Check sheet for the modelled part. Datum: model origin and axes. Units: mm. A direction names the side the tool comes from. Give positions to 0.01 mm unless a question says otherwise; leave off trailing zeros. Write each loop counter-clockwise with the first axis right and the second up, starting at its lowest first coordinate (ties: lowest second). Pieces come first, ordered by that corner, then holes. Notation, with made-up numbers: M 4.5,85 L 44.5,85 A15 cw 44.5,90 Z; hole C 78,-8 d4. An arc over 180 degrees is marked long. Use CSV: the item, a comma, the result in double quotes. Start each with the question number.
1. Cross-section at D-D, the plane x = 5.5. Enter the section's corners in (y, z).
2. Access from +Z, -Z, +X, -X, +Y, -Y to the whole of each face (thin tool, end or side, straight path). Record for faces 1 (the face through (-6, 10, -2)), 2 (the face through (0, 3, -2.975)), 3 (the face through (2.975, 3, 0)), 4 (the face through (0, 3, 2.975)), 5 (the face through (-2.777, 7.972, 6.697)).
3. Depth check by flat-ended pin: P1, Ø4.5, axis at x = 3, z = 0, coming from the -Y side; P2, Ø1.7, axis at x = 0, z = 0, coming from the -Y side; P3, Ø4, axis at y = 9.5, z = 4.5, coming from the -X side; P4, Ø4, axis at x = -3.5, y = 3, coming from the +Z side (3 decimals). Enter the tip coordinate at first touch or a pass-through.
4. Cross-section at C-C, the plane z = -5. Enter the section's corners in (x, y).
5. Cross-section at B-B, the plane x = -0.25. Enter the section's corners in (y, z) (3 decimals), and give its area (3 significant figures).
6. Cross-section at A-A, the plane y = 3.75. Enter the section's corners in (x, z) (3 decimals).
7. Scan lines: line 1 (Z direction, x = 0, y = 3.25) (3 decimals); line 2 (X direction, y = 8, z = 0) (3 decimals). Record each from-to range of solid material in increasing order.
8. Mould release check, pull along X, two halves, no side actions. Record for faces 6 (the face through (0, 12.2, -5.5)), 7 (the face through (-2.975, 3, 0)), 8 (the face through (0.1, 6, -3.3)): +X half, -X half, draft (parallel to the pull), parting line (faces both ways), or undercut.
from build123d import *

# Parameters (mm, degrees)
SKETCH1_W           = 5.95
SKETCH1_H           = 5.95
BOSS_EXTRUDE1_DEPTH = 6
SKETCH2_R           = 7.25
BOSS_EXTRUDE2_DEPTH = 4
SKETCH3_R           = 1.425
CUT_EXTRUDE1_DEPTH  = 15.322185587
SKETCH4_R           = 1.425
BOSS_EXTRUDE4_DEPTH = 4.5


with BuildPart() as part:
    # Sketch1 → Boss-Extrude1 (new body)
    with BuildSketch(Plane(origin=(0, 0, 0), x_dir=(1, 0, 0), z_dir=(0, 1, 0))):
        Rectangle(SKETCH1_W, SKETCH1_H)
    extrude(amount=BOSS_EXTRUDE1_DEPTH)

    # Sketch2 → Boss-Extrude2 (add)
    with BuildSketch(Plane(origin=(0, 6, 0), x_dir=(1, 0, 0), z_dir=(0, 1, 0))):
        with Locations(Location((0, 0, 0), (0, 0, 270))):
            Circle(SKETCH2_R)
    extrude(amount=BOSS_EXTRUDE2_DEPTH)

    # Sketch3 → Cut-Extrude1 (cut, through all)
    with BuildSketch(Plane.XZ):
        with Locations(Location((0, 0, 0), (0, 0, 270))):
            Circle(SKETCH3_R)
    extrude(amount=-CUT_EXTRUDE1_DEPTH, mode=Mode.SUBTRACT)

    # Sketch4 → Boss-Extrude4 (add)
    with BuildSketch(Plane(origin=(0, 10, 0), x_dir=(1, 0, 0), z_dir=(0, 1, 0))):
        with BuildLine():
            ThreePointArc((-0.499565784, 5.979166667), (-4.062179544, -4.415732935), (6, 0))
            ThreePointArc((6, 0), (4.415732935, 4.062179544), (0.499565784, 5.979166667))
            ThreePointArc((0.499565784, 5.979166667), (0, 5.5), (-0.499565784, 5.979166667))
        make_face()
        with Locations(Location((0, 0, 0), (0, 0, 90))):
            Circle(SKETCH4_R, mode=Mode.SUBTRACT)
    extrude(amount=BOSS_EXTRUDE4_DEPTH)


solid = part.part
Worked answers:
1,outline,"M 6,-4.72 L 10,-4.72 L 10,-2.4 L 14.5,-2.4 L 14.5,2.4 L 10,2.4 L 10,4.72 L 6,4.72 Z"
2,face 1,"+Y"
2,face 2,"-Z, +X, -X, -Y"
2,face 3,"+Z, -Z, +X, -Y"
2,face 4,"+Z, +X, -X, -Y"
2,face 5,"+Y, -Y"
3,P1,"stops at y = 0"
3,P2,"passes through"
3,P3,"stops at x = -6.81"
3,P4,"stops at z = 2.975"
4,outline,"M -5.25,6 L 5.25,6 L 5.25,10 L 3.32,10 L 3.32,14.5 L -3.32,14.5 L -3.32,10 L -5.25,10 Z"
5,outline,"M 0,-2.975 L 6,-2.975 L 6,-7.246 L 10,-7.246 L 10,-5.567 L 14.5,-5.567 L 14.5,-1.403 L 0,-1.403 Z; M 0,1.403 L 14.5,1.403 L 14.5,5.995 L 10,5.995 L 10,7.246 L 6,7.246 L 6,2.975 L 0,2.975 Z"
5,area,"105 mm^2"
6,outline,"M -2.975,-2.975 L 2.975,-2.975 L 2.975,2.975 L -2.975,2.975 Z; hole C 0,0 d2.85"
7,line 1,"z = -2.975 to -1.425, 1.425 to 2.975"
7,line 2,"x = -7.25 to -1.425, 1.425 to 7.25"
8,face 6,"undercut"
8,face 7,"-X half"
8,face 8,"draft"
